Autodesk Inventor part; units mm, degrees
ref_plane "YZ Plane" through (0, 0, 0) normal (1, 0, 0) x (0, 1, 0)
ref_plane "XZ Plane" through (0, 0, 0) normal (0, 1, 0) x (-1, 0, 0)
ref_plane "XY Plane" through (0, 0, 0) normal (0, 0, 1) x (1, 0, 0)
sketch "Boceto1" plane through (0, 0, 0) normal (0, 0, 1) x (1, 0, 0)
  circle A0 centre (0, 0) radius 13.31
  dimension "d0" = 26.62
extrude "Extrusión1" add sketch "Boceto1" along normal mid plane 21.54
sketch "Boceto2" plane through (0, 0, 0) normal (0, 1, 0) x (-1, 0, 0)
  point P0 (0, 0)
hole "Hole1" at (0, 0, 10.77) direction (0, 0, -1) diameter 10.78 depth 0.8
hole "Hole2" at (0, 0, -10.77) direction (0, 0, 1) diameter 25.82 depth 20.74
fillet "Empalme1" radius 2 1 edges at (-13.31, 0, 10.77)
properties part number "CajaMotor"
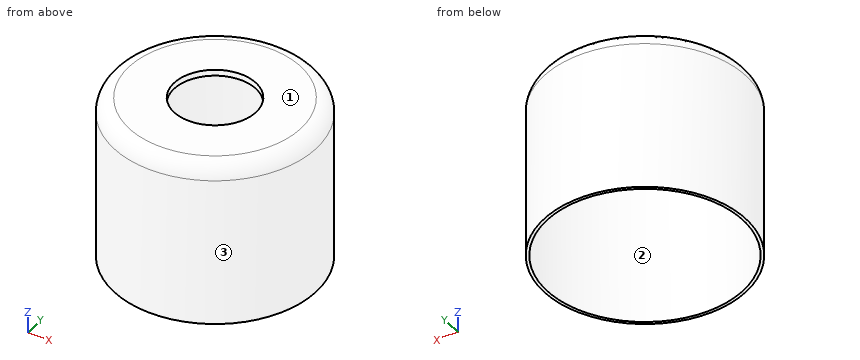
Read the model definition and answer for the solid it produces. Units are mm, in the model's axes. Face numbers are marked on the shaded views. Round coordinates to 2 decimals unless told otherwise and drop trailing zeros. Write each loop counter-clockwise with the first axis right and the second up, starting at its lowest first coordinate (ties: lowest second). Pieces come first, ordered by that corner, then holes.
1. Straight lines are drawn through the part: L1, parallel to Y at x = 0, z = -5.25; L2, parallel to Z at x = -1.75, y = 6.75; L3, parallel to Y at x = -3.25, z = 2.5. For each, find the intervals that lie inside material, in ascending order.
2. Determine the mould class of the marked faces 1, 2 and 3 for opening direction Y: pulls with the +Y half, pulls with the -Y half, needs draft (parallel to the pull), parting line crosses it, or undercut.
3. The part is cut by section C-C, the plane z = -8. Determine the outline of the cut face in (x, y).
4. Given pin 1 Ø3 at (y, z) = (8, -2) entering from +X; pin 2 Ø1.5 at (y, z) = (2, 8.5) entering from +X; pin 3 Ø3 at (y, z) = (10, 0.5) entering from -X, each flat-ended and moving along its own axis, determine where each tip first touches the part or whether it passes through.
Values:
1. L1: y = -13.31 to -12.91, 12.91 to 13.31
1. L2: z = 9.97 to 10.77
1. L3: y = -12.91 to -12.49, 12.49 to 12.91
2. face 1: needs draft
2. face 2: undercut
2. face 3: parting line crosses it
3. outline: circle Ø26.62 at (0, 0); hole circle Ø25.82 at (0, 0)
4. pin 1: stops at x = 11.61
4. pin 2: stops at x = 13.25
4. pin 3: stops at x = -10.24
